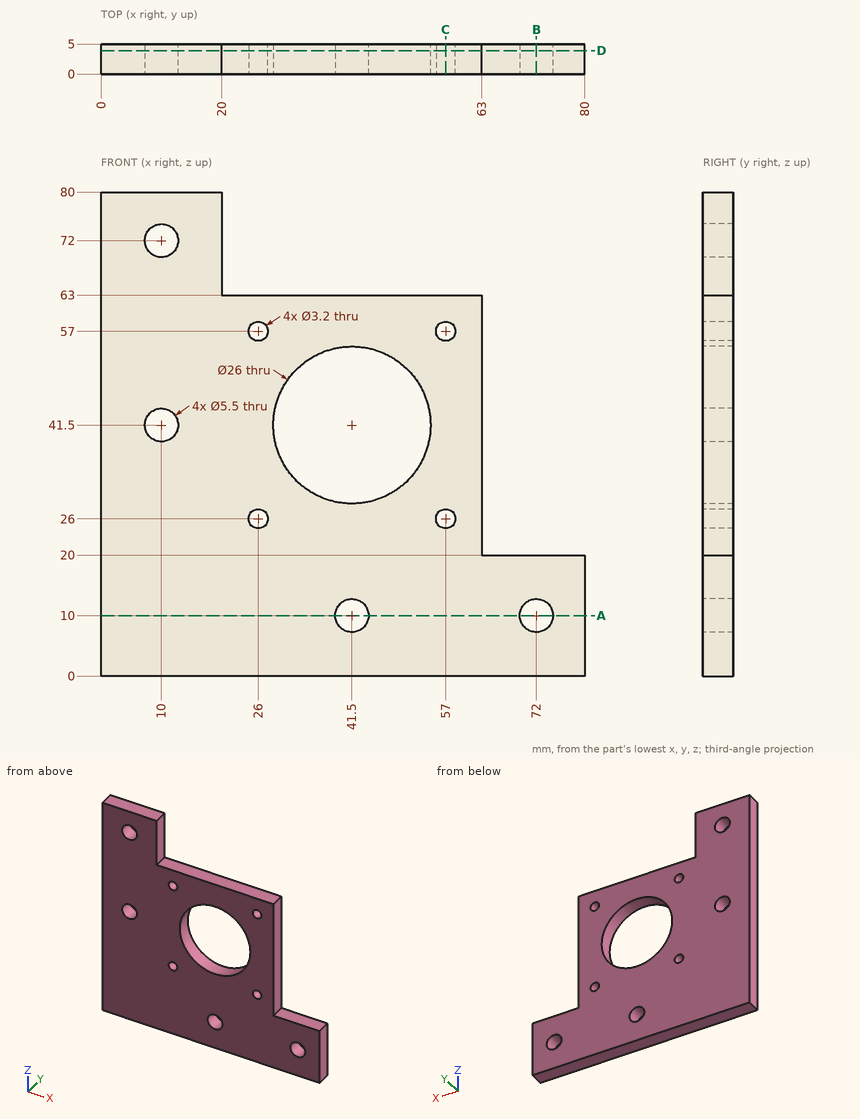
Geometry: see drawing. Coordinates: mm, zero at the bounding-box minimum. Coordinates: 2 decimals unless noted, no trailing zeros. Loops run counter-clockwise (first coordinate to the right, second up) from the corner with the lowest first, then second, coordinate; pieces in that order, holes last.
(1) Section B-B on x = 72. Return the cut outline in (y, z), then the cut area to 3 significant figures.
(2) First-contact query: pin 1 Ø3.5 at (x, z) = (10, 41.5) entering from -Y; pin 2 Ø2.5 at (x, y) = (42.5, 1.5) entering from +Z; pin 3 Ø1.5 at (y, z) = (2.5, 49) entering from +X. Flat tips, straight axial feed; report the tip coordinate or a pass-through.
(3) Section D-D on y = 3.9. Count the separate pieces of the cut face and the enclosed holes in it, then the cut area to 3 significant figures.
(4) Material intervals for probe 1 along Z at (x, y) = (10, 1.45); probe 2 along X at (y, z) = (3.3, 41.5), sorted ascending.
(5) Section A-A on z = 10. Return the cut outline in (x, y), then the cut area to 3 significant figures.
(6) Section C-C on x = 57. Return the cut outline in (y, z), then the cut area to 3 significant figures.
Data:
1. outline: (0, 0) - (5, 0) - (5, 7.25) - (0, 7.25) - close; (0, 12.75) - (5, 12.75) - (5, 20) - (0, 20) - close
1. area: 72.5 mm2
2. pin 1: passes through
2. pin 2: stops at z = 63
2. pin 3: stops at x = 63
3. separate pieces: 1
3. enclosed holes: 9
3. area: 3,990 mm2
4. probe 1: z = 0 to 38.75, 44.25 to 69.25, 74.75 to 80
4. probe 2: x = 0 to 7.25, 12.75 to 28.5, 54.5 to 63
5. outline: (0, 0) - (38.75, 0) - (38.75, 5) - (0, 5) - close; (44.25, 0) - (69.25, 0) - (69.25, 5) - (44.25, 5) - close; (74.75, 0) - (80, 0) - (80, 5) - (74.75, 5) - close
5. area: 345 mm2
6. outline: (0, 0) - (5, 0) - (5, 24.4) - (0, 24.4) - close; (0, 27.6) - (5, 27.6) - (5, 55.4) - (0, 55.4) - close; (0, 58.6) - (5, 58.6) - (5, 63) - (0, 63) - close
6. area: 283 mm2
